Could you check a few things on this model? Use its own coordinates, in mm. Face numbers are marked on the shaded views. A direction names the side the tool comes from. Give positions to 0.01 mm unless a question says otherwise; leave off trailing zeros. Loops run counter-clockwise (first coordinate to the right, second up) from the corner with the lowest first, then second, coordinate; pieces in that order, holes last. Notation, with made-up numbers: M -35,-26 L -29,-26 A27 ccw -29,-2 Z; hole C -17.75,-25 d8. An arc over 180 degrees is marked long. Use a Markdown table: item, result. Add a question column.
1) Suppose I cut it at C-C on y = -3.5. List the corners of the cut face in (x, z) for me.
2) Suppose I cut it at D-D on z = 7. List the corners of the cut face in (x, y) for me.
3) We'd pull the mould along Y, two halves only. Please class the marked faces 1, 2, 3 and 4: +Y half, -Y half, draft (parallel to the pull), parting line (faces both ways), or undercut.
4) Suppose I cut it at B-B on x = -17.5. List the corners of the cut face in (y, z) for me, and give its area (3 significant figures).
5) Will these pins go through, and if not, where does the flat tip stop? pin 1 Ø6 at (y, z) = (12.5, 2.5) entering from -X; pin 2 Ø2 at (x, z) = (-3, 7) entering from +Y; pin 3 Ø9.5 at (x, z) = (-18.5, 6.5) entering from -Y; pin 4 Ø1.5 at (x, y) = (-12, 6.5) entering from +Z.
6) If I drill on line 1 along Y through (x, z) = (-37.5, -14); line 2 along X through (y, z) = (-17.5, 0.5); line 3 along Y through (x, z) = (-32.5, -5.5), over which ranges is the centre line in solid material (lowest first)? Write a range as [from, to].
7) Suppose I cut it at A-A on z = -11.5. List the corners of the cut face in (x, y) for me.
8) Which directions (+Z, -Z, +X, -X, +Y, -Y) give clear straight access to the entire face, cutting with the end or side of a thin tool? Please do the marked faces 5 and 6.
```python
from build123d import *

# Parameters (mm, degrees)
F0_W      = 10
F0_H      = 23.902074
F1_DEPTH  = 1.2
F2_DEPTH  = 10
F0_R      = 2.65
F3_DEPTH  = 10
F4_DEPTH  = 26
F5_W      = 18
F5_H      = 8
F6_DEPTH  = 3
F7_W      = 9.7
F7_H      = 8
F8_DEPTH  = 25
F9_W      = 5
F9_H      = 3
F10_DEPTH = 4


with BuildPart() as f1:
    # F0 (on Top) → F1 (new body)
    with BuildSketch(Plane.XY):
        Polygon((-31.738877, -7.347546), (-31.738877, -17.747546), (-3.738877, -17.747546), (-3.738877, -7.347546), (-5.738877, -7.347546), (-5.738877, 2.652454), (-3.738877, 2.652454), (-3.738877, 13.052454), (-31.738877, 13.052454), (-31.738877, 2.652454), (-29.738877, 2.652454), (-29.738877, -7.347546), align=None)
        with Locations((-17.738877, -2.347546)):
            Rectangle(F0_W, F0_H, mode=Mode.SUBTRACT)
    extrude(amount=F1_DEPTH)

    # F0 (on Top) → F2 (join)
    with BuildSketch(Plane.XY):
        with BuildLine():
            Line((-3.738877, -17.747546), (-31.738877, -17.747546))
            ThreePointArc((-31.738877, -17.747546), (-31.844346, -18.769095), (-32.156302, -19.747546))
            Line((-32.156302, -19.747546), (-1.738877, -19.747546))
            Line((-1.738877, -19.747546), (-1.738877, 15.052454))
            Line((-1.738877, 15.052454), (-32.156302, 15.052454))
            ThreePointArc((-32.156302, 15.052454), (-31.844346, 14.074002), (-31.738877, 13.052454))
            Line((-31.738877, 13.052454), (-3.738877, 13.052454))
            Line((-3.738877, 13.052454), (-3.738877, 2.652454))
            Line((-3.738877, 2.652454), (-3.738877, -7.347546))
            Line((-3.738877, -7.347546), (-3.738877, -17.747546))
        make_face()
        with BuildLine():
            ThreePointArc((-33.738877, -13.747546), (-32.266741, -15.511478), (-31.738877, -17.747546))
            Line((-31.738877, -17.747546), (-31.738877, -7.347546))
            Line((-31.738877, -7.347546), (-31.738877, 2.652454))
            Line((-31.738877, 2.652454), (-31.738877, 13.052454))
            ThreePointArc((-31.738877, 13.052454), (-32.266741, 10.816386), (-33.738877, 9.052454))
            Line((-33.738877, 9.052454), (-33.738877, -13.747546))
        make_face()
        with BuildLine():
            Line((-33.738877, 15.052454), (-33.738877, 9.052454))
            ThreePointArc((-33.738877, 9.052454), (-32.266741, 10.816386), (-31.738877, 13.052454))
            ThreePointArc((-31.738877, 13.052454), (-31.844346, 14.074002), (-32.156302, 15.052454))
            Line((-32.156302, 15.052454), (-33.738877, 15.052454))
        make_face()
        with BuildLine():
            ThreePointArc((-32.156302, -19.747546), (-31.844346, -18.769095), (-31.738877, -17.747546))
            ThreePointArc((-31.738877, -17.747546), (-32.266741, -15.511478), (-33.738877, -13.747546))
            Line((-33.738877, -13.747546), (-33.738877, -19.747546))
            Line((-33.738877, -19.747546), (-32.156302, -19.747546))
        make_face()
    extrude(amount=F2_DEPTH)

    # F0 (on Top) → F3 (join)
    with BuildSketch(Plane.XY):
        with BuildLine():
            ThreePointArc((-32.156302, 15.052454), (-41.57353, 14.327654), (-33.738877, 9.052454))
            Line((-33.738877, 9.052454), (-33.738877, 15.052454))
            Line((-33.738877, 15.052454), (-32.156302, 15.052454))
        make_face()
        with Locations((-36.738877, 13.052454)):
            Circle(F0_R, mode=Mode.SUBTRACT)
        with BuildLine():
            Line((-33.738877, -19.747546), (-33.738877, -13.747546))
            ThreePointArc((-33.738877, -13.747546), (-41.57353, -19.022747), (-32.156302, -19.747546))
            Line((-32.156302, -19.747546), (-33.738877, -19.747546))
        make_face()
        with Locations((-36.738877, -17.747546)):
            Circle(F0_R, mode=Mode.SUBTRACT)
    extrude(amount=F3_DEPTH)

    # F0 (on Top) → F4 (join)
    with BuildSketch(Plane.XY):
        with BuildLine():
            ThreePointArc((-32.156302, 15.052454), (-41.57353, 14.327654), (-33.738877, 9.052454))
            Line((-33.738877, 9.052454), (-33.738877, 15.052454))
            Line((-33.738877, 15.052454), (-32.156302, 15.052454))
        make_face()
        with Locations((-36.738877, 13.052454)):
            Circle(F0_R, mode=Mode.SUBTRACT)
        with BuildLine():
            Line((-33.738877, 15.052454), (-33.738877, 9.052454))
            ThreePointArc((-33.738877, 9.052454), (-32.266741, 10.816386), (-31.738877, 13.052454))
            ThreePointArc((-31.738877, 13.052454), (-31.844346, 14.074002), (-32.156302, 15.052454))
            Line((-32.156302, 15.052454), (-33.738877, 15.052454))
        make_face()
        with BuildLine():
            Line((-33.738877, -19.747546), (-33.738877, -13.747546))
            ThreePointArc((-33.738877, -13.747546), (-41.57353, -19.022747), (-32.156302, -19.747546))
            Line((-32.156302, -19.747546), (-33.738877, -19.747546))
        make_face()
        with Locations((-36.738877, -17.747546)):
            Circle(F0_R, mode=Mode.SUBTRACT)
        with BuildLine():
            ThreePointArc((-32.156302, -19.747546), (-31.844346, -18.769095), (-31.738877, -17.747546))
            ThreePointArc((-31.738877, -17.747546), (-32.266741, -15.511478), (-33.738877, -13.747546))
            Line((-33.738877, -13.747546), (-33.738877, -19.747546))
            Line((-33.738877, -19.747546), (-32.156302, -19.747546))
        make_face()
    extrude(amount=-F4_DEPTH)

    # F5 (on face) → F6 (cut)
    with BuildSketch(Plane.YZ.offset(-1.738877)):
        with Locations((-8.747546, 6)):
            Rectangle(F5_W, F5_H)
    extrude(amount=-F6_DEPTH, mode=Mode.SUBTRACT)

    # F7 (on face) → F8 (cut)
    with BuildSketch(Plane.XZ.offset(-13.052454)):
        with Locations((-26.888877, 6)):
            Rectangle(F7_W, F7_H)
    extrude(amount=-F8_DEPTH, mode=Mode.SUBTRACT)

    # F9 (on face) → F10 (cut)
    with BuildSketch(Plane(origin=(-33.738877, 0, 0), x_dir=(0, -1, 0), z_dir=(-1, 0, 0))):
        with Locations((-1.652454, 3.7)):
            Rectangle(F9_W, F9_H)
    extrude(amount=-F10_DEPTH, mode=Mode.SUBTRACT)


solid = f1.part
```
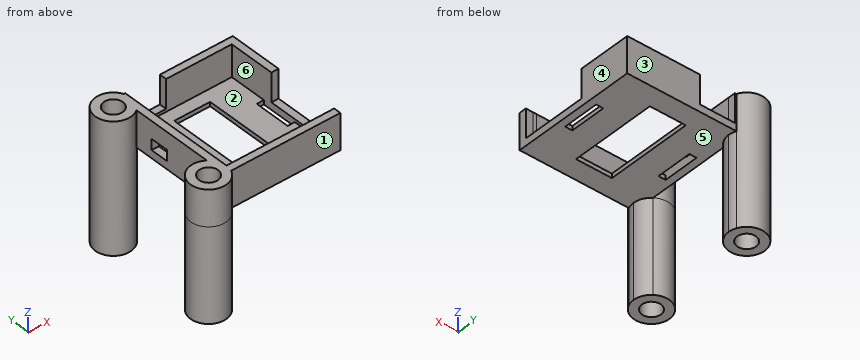
Answer block:
| question | item | result |
|---|---|---|
| 1 | outline | M -33.74,0 L -31.74,0 L -31.74,10 L -33.74,10 Z; M -29.74,0 L -22.74,0 L -22.74,1.2 L -29.74,1.2 Z; M -12.74,0 L -5.74,0 L -5.74,1.2 L -12.74,1.2 Z; M -3.74,0 L -1.74,0 L -1.74,2 L -3.74,2 Z |
| 2 | outline | M -33.74,-13.75 A5 ccw long -32.16,-19.75 L -1.74,-19.75 L -1.74,-17.75 L -31.74,-17.75 L -31.74,15.05 L -32.16,15.05 A5 ccw long -33.74,9.05 Z; M -22.04,13.05 L -3.74,13.05 L -3.74,0.25 L -1.74,0.25 L -1.74,15.05 L -22.04,15.05 Z; hole C -36.74,-17.75 d5.3; hole C -36.74,13.05 d5.3 |
| 3 | face 1 | -Y half |
| 3 | face 2 | undercut |
| 3 | face 3 | +Y half |
| 3 | face 4 | draft |
| 4 | outline | M -19.75,0 L -14.3,0 L -14.3,1.2 L -17.75,1.2 L -17.75,10 L -19.75,10 Z; M 9.6,0 L 15.05,0 L 15.05,10 L 13.05,10 L 13.05,1.2 L 9.6,1.2 Z |
| 4 | area | 48.3 mm^2 |
| 5 | pin 1 | stops at x = -41.74 |
| 5 | pin 2 | stops at y = 15.05 |
| 5 | pin 3 | stops at y = -19.75 |
| 5 | pin 4 | stops at z = 1.2 |
| 6 | line 1 | y = [-22.69, -20.29], [-15.21, -12.81], [8.11, 10.51], [15.59, 17.99] |
| 6 | line 2 | x = [-41.73, -39.38], [-34.1, -1.74] |
| 6 | line 3 | y = [-20.4, -15.1], [10.4, 15.7] |
| 7 | outline | M -33.74,-13.75 A5 ccw long -32.16,-19.75 A5 ccw -31.74,-17.75 A5 ccw Z; M -32.16,15.05 A5 ccw long -31.74,13.05 A5 ccw Z; hole C -36.74,-17.75 d5.3; hole C -36.74,13.05 d5.3 |
| 8 | face 5 | -Z, +X |
| 8 | face 6 | +Z |
